from build123d import *

# Parameters (mm, degrees)
F1_DEPTH = 228.6
F2_T     = -7.257143


with BuildPart() as f1:
    # F0 (on Front) → F1 (new body)
    with BuildSketch(Plane.XZ):
        Polygon((-74.641859, 25.4), (-74.641859, -25.4), (-44.782368, -66.498063), (3.531303, -82.196127), (51.844974, -66.498063), (81.704465, -25.4), (81.704465, 25.4), (51.844974, 66.498063), (3.531303, 82.196127), (-44.782368, 66.498063), align=None)
    extrude(amount=F1_DEPTH)

    # F2
    f2_openings = [f1.faces().sort_by_distance(p)[0] for p in [
        (3.531303, -228.6, 0),
    ]]
    offset(amount=F2_T, openings=f2_openings)


solid = f1.part
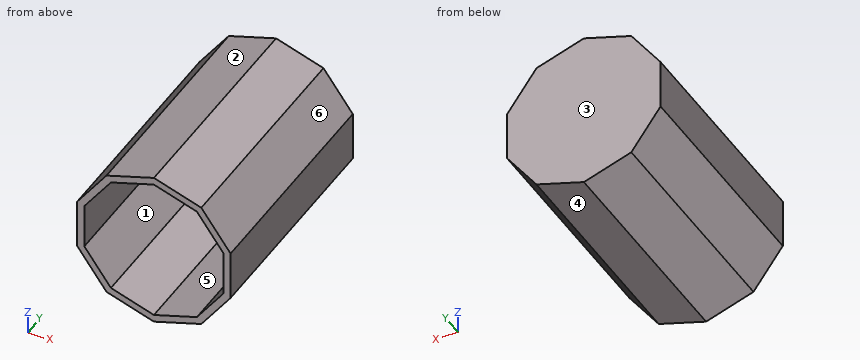
Design review of the part built by this model. Coordinates are the model's own, in mm. Face numbers are marked on the shaded views. A direction names the side the tool comes from. Coordinates: 2 decimals unless noted, no trailing zeros. Order: outer loops, then holes, each group sorted by start corner. A loop starts at its lowest first (then second) coordinate and runs counter-clockwise, first axis right, second up. Notation, with made-up numbers: (-24, -34) - (29, -34) arc R27 cw to (29, -16) - close; hole circle Ø8 at (-24, 54.5). An arc over 180 degrees is marked (long way). Put each result on its own line as item: value.
1) Take a section at B-B, the plane z = -7. Give the boundary of the cut face in (x, y).
Response values:
outline: (-74.64, -228.6) - (-67.38, -228.6) - (-67.38, -7.26) - (74.45, -7.26) - (74.45, -228.6) - (81.7, -228.6) - (81.7, 0) - (-74.64, 0) - close
2) Tool access review of the marked faces 5 and 6: name each direction out of +Z, -Z, +X, -X, +Y, -Y from which nothing blocks a thin tool from reaching the whole face with its end or side.
Response values:
face 5: -Y
face 6: +Z, +X, +Y, -Y
3) Take a section at C-C, the plane x = 41. Give the boundary of the cut face in (y, z).
Response values:
outline: (-228.6, -70.02) - (0, -70.02) - (0, 70.02) - (-228.6, 70.02) - (-228.6, 62.39) - (-7.26, 62.39) - (-7.26, -62.39) - (-228.6, -62.39) - close
4) Insertion check: P1, Ø12, axis at x = -54, y = -28, coming from the +Z side; P2, Ø4, axis at y = -181, z = -40.5, coming from the -X side; P3, Ø4, axis at x = -43, z = -46.5, coming from the -Y side. Each pin has a flat end and moves straight along its axis. Give the tip position at first contact, or say it passes through.
Response values:
P1: stops at z = 62.07
P2: stops at x = -65.12
P3: stops at y = -7.26
5) Wall thickness on L1, parallel to X at y = -84, z = 3; L2, parallel to Y at x = -26, z = -20; L3, parallel to Z at x = -37, y = -23.5: over which ranges is each line inside the solid? List them lowest first. Write a range as from..to.
Response values:
L1: x = -74.64..-67.38, 74.45..81.7
L2: y = -7.26..0
L3: z = -69.03..-61.4, 61.4..69.03
6) Take a section at A-A, the plane y = -106. Give the boundary of the cut face in (x, z).
Response values:
outline: (-74.64, -25.4) - (-44.78, -66.5) - (3.53, -82.2) - (51.84, -66.5) - (81.7, -25.4) - (81.7, 25.4) - (51.84, 66.5) - (3.53, 82.2) - (-44.78, 66.5) - (-74.64, 25.4) - close; hole (-67.38, -23.04) - (-40.3, -60.32) - (3.53, -74.57) - (47.36, -60.32) - (74.45, -23.04) - (74.45, 23.04) - (47.36, 60.32) - (3.53, 74.57) - (-40.3, 60.32) - (-67.38, 23.04) - close
7) The part is to be moulded in two halves that separate along X. For the marked faces 1, 2, 3 and 4, say which applies: released by +X, released by -X, zero draft, split by the parting line, or undercut.
Response values:
face 1: undercut
face 2: released by -X
face 3: zero draft
face 4: released by +X
